```python
from build123d import *

# Parameters (mm, degrees)
BOSS_EXTRUDE4_DEPTH = 4
BOSS_EXTRUDE6_DEPTH = 5
CUT_EXTRUDE1_REACH  = 22.155
CUT_EXTRUDE2_REACH  = 22.155
SKETCH9_R           = 3


with BuildPart() as part:
    # Sketch1 → Boss-Extrude4 (new body)
    with BuildSketch(Plane.XY):
        Polygon((0, 0), (8.226600985, 5), (8.226600985, 0), align=None)
    extrude(amount=BOSS_EXTRUDE4_DEPTH)

    # Sketch7 → Boss-Extrude6 (add)
    with BuildSketch(Plane(origin=(0, 0, 0), x_dir=(1, 0, 0), z_dir=(0, 1, 0))):
        with BuildLine():
            Line((13.226600985, 3), (4.113300493, 0))
            Line((4.113300493, 0), (8.226600985, 0))
            Line((8.226600985, 0), (8.226600985, -4))
            Line((8.226600985, -4), (4.113300493, -4))
            Line((4.113300493, -4), (13.226600985, -7))
            ThreePointArc((13.226600985, -7), (18.226600985, -2), (13.226600985, 3))
        make_face()
    extrude(amount=BOSS_EXTRUDE6_DEPTH)

    # Sketch8 → Cut-Extrude1 (cut, up to next)
    with BuildSketch(Plane.XY, mode=Mode.PRIVATE) as cut_extrude1_sk1:
        Polygon((4.113300493, 2.5), (4.113300493, 5), (8.226600985, 5), align=None)
    cut_extrude1_tool1 = extrude(cut_extrude1_sk1.sketch, amount=-CUT_EXTRUDE1_REACH, mode=Mode.PRIVATE) & part.part
    cut_extrude1 = cut_extrude1_tool1.solids().sort_by_distance((5.484401, 4.166667, 0))[0]
    add(cut_extrude1, mode=Mode.SUBTRACT)

    # Mirror1: Cut-Extrude1 across plane
    add(cut_extrude1.mirror(Plane.XY.offset(2)), mode=Mode.SUBTRACT)

    # Sketch9 → Cut-Extrude2 (cut, up to next)
    with BuildSketch(Plane(origin=(0, 5, 0), x_dir=(1, 0, 0), z_dir=(0, 1, 0)), mode=Mode.PRIVATE) as cut_extrude2_sk1:
        with Locations(Location((13.226600985, -2, 0), (0, 0, 270))):
            Circle(SKETCH9_R)
    cut_extrude2_tool1 = extrude(cut_extrude2_sk1.sketch, amount=-CUT_EXTRUDE2_REACH, mode=Mode.PRIVATE) & part.part
    add(cut_extrude2_tool1.solids().sort_by_distance((13.226601, 5, 2))[0], mode=Mode.SUBTRACT)


solid = part.part
```
CAD build for the part. Positions are in the model's coordinates, mm. Coordinates: 2 decimals unless noted, no trailing zeros. Loops run counter-clockwise (first coordinate to the right, second up) from the corner with the lowest first, then second, coordinate; pieces in that order, holes last. Notation, with made-up numbers: (6.25, 38.5) - (16.25, 38.5) arc R25 cw to (16.25, 65.5) - close; hole circle Ø10 at (61.5, -27.75). An arc over 180 degrees is marked (long way). Return JSON: item names as keys, results as strings.
1. Mould opens along Z. For faces 1 (the cylindrical face through (16.2, 2.5, 1.6)), 2 (the flat face through (9, 0, 2)), 3 (the flat face through (3, 1, 0)), 4 (the flat face through (3, 1, 4)) say: released by +Z, released by -Z, zero draft, split by the parting line, or undercut.
Result:
{"face 1": "undercut", "face 2": "zero draft", "face 3": "released by -Z", "face 4": "released by +Z"}
2. Drop flat-ended pins along their axis: pin 1 (6 mm diameter, centred on x = 3, z = 1, fed in from -Y); pin 2 (5.5 mm diameter, centred on x = 13.23, z = 2, fed in from -Y); pin 3 (3 mm diameter, centred on x = 9, y = 3, fed in from +Z); pin 4 (1.3 mm diameter, centred on x = 1.5, y = 1, fed in from -Z). Give the stop position or say it passes through.
Result:
{"pin 1": "stops at y = 0", "pin 2": "passes through", "pin 3": "stops at z = 6.1", "pin 4": "stops at z = 0"}
3. Band-saw the part on A-A (z = 2). Give the cut face in (x, y), and give its area (3 significant figures).
Result:
{"outline": "(0, 0) - (10.23, 0) - (10.23, 5) - (8.23, 5) - close; (16.23, 0) - (18.23, 0) - (18.23, 5) - (16.23, 5) - close", "area": "40.6 mm2"}
4. Band-saw the part on D-D (y = 3.5). Give the cut face in (x, z), and give its area (3 significant figures).
Result:
{"outline": "(5.76, -0.54) - (13.23, -3) arc R5 ccw to (13.23, 7) - (5.76, 4.54) - close; hole circle Ø6 at (13.23, 2)", "area": "67.3 mm2"}
5. Probe L1, parallel to Z at x = 2.5, y = 1.35; L2, parallel to X at y = 2.6, z = 2; L3, parallel to X at y = 3.55, z = 2.5. List the from-to ranges inside material, lowest first. Write a range as from..to.
Result:
{"L1": "z = 0..4", "L2": "x = 4.28..10.23, 16.23..18.23", "L3": "x = 5.84..10.27, 16.18..18.2"}
6. Band-saw the part on C-C (z = -0.75). Give the cut face in (x, y).
Result:
{"outline": "(6.39, 0) - (12.03, 0) - (12.03, 5) - (8.23, 5) - (6.39, 3.88) - close; (14.43, 0) - (17.4, 0) - (17.4, 5) - (14.43, 5) - close"}
7. Band-saw the part on B-B (y = 1.8). Give the cut face in (x, z), and give its area (3 significant figures).
Result:
{"outline": "(2.96, 0) - (4.11, 0) - (13.23, -3) arc R5 ccw to (13.23, 7) - (4.11, 4) - (2.96, 4) - close; hole circle Ø6 at (13.23, 2)", "area": "79.4 mm2"}
